```python
from build123d import *

# Parameters (mm, degrees)
F0_R     = 12.7
F0_R_2   = 9.144
F0_R_3   = 2.794
F1_DEPTH = 69.85
F2_DEPTH = 69.851
F3_DEPTH = 19.05


with BuildPart() as f1:
    # F0 (on Top) → F1 (new body)
    with BuildSketch(Plane.XY):
        Circle(F0_R)
        Circle(F0_R_2, mode=Mode.SUBTRACT)
        Circle(F0_R_2)
        Circle(F0_R_3, mode=Mode.SUBTRACT)
        Circle(F0_R_3)
    extrude(amount=F1_DEPTH)

    # F0 (on Top) → F2 (cut, through all)
    with BuildSketch(Plane.XY):
        Circle(F0_R_3)
    extrude(amount=F2_DEPTH, mode=Mode.SUBTRACT)

    # F0 (on Top) → F3 (cut)
    with BuildSketch(Plane.XY):
        Circle(F0_R_2)
        Circle(F0_R_3, mode=Mode.SUBTRACT)
    extrude(amount=F3_DEPTH, mode=Mode.SUBTRACT)


solid = f1.part
```
Can you work these out from the model? Positions are in its coordinate system, mm. A direction names the side the tool comes from. Round coordinates to 2 decimals unless told otherwise and drop trailing zeros. Loops run counter-clockwise (first coordinate to the right, second up) from the corner with the lowest first, then second, coordinate; pieces in that order, holes last.
Item 1: Suppose I cut it at C-C, the plane x = 7.5. Write out the boundary of the cut face in (y, z), then the cut area to 3 significant figures.
Item 2: Will these pins go through, and if not, where does the flat tip stop? pin 1 Ø4 at (x, z) = (9.5, 34.5) entering from +Y; pin 2 Ø4 at (y, z) = (9.5, 51.5) entering from +X; pin 3 Ø1.5 at (y, z) = (-9.5, 15.5) entering from -X.
Item 3: Please list where these lines run through material, in increasing order: L1, parallel to Y at x = 0, z = 7; L2, parallel to Y at x = 0, z = 49; L3, parallel to Z at x = 1, y = 8.5.
Item 4: Which directions (+Z, -Z, +X, -X, +Y, -Y) give clear straight access to the entire face, cutting with the end or side of a thin tool? Please do faces 1 (the cylindrical face through (-2.217, -1.7, 44.094)), 2 (the cylindrical face through (-1.982, -8.927, 9.392)).
Item 5: If we mould it in two halves opening along X, with no side actions, what happens to faces 3 (the flat face through (-9, 3, 0)), 4 (the flat face through (-2.2, 2.2, 19.05)), 5 (the cylindrical face through (-2.75, -12.4, 34.44))? For each: +X half, -X half, draft (parallel to the pull), parting line (faces both ways), or undercut.
Item 6: Suppose I cut it at D-D, the plane z = 49. Write out the boundary of the cut face in (x, y).
Item 7: Suppose I cut it at A-A, the plane y = 0. Write out the boundary of the cut face in (x, z).
Reported:
1. outline: (-10.25, 0) - (-5.23, 0) - (-5.23, 19.05) - (5.23, 19.05) - (5.23, 0) - (10.25, 0) - (10.25, 69.85) - (-10.25, 69.85) - close
1. area: 1,230 mm2
2. pin 1: stops at y = 10.25
2. pin 2: stops at x = 10.25
2. pin 3: stops at x = -9.2
3. L1: y = -12.7 to -9.14, 9.14 to 12.7
3. L2: y = -12.7 to -2.79, 2.79 to 12.7
3. L3: z = 19.05 to 69.85
4. face 1: +Z, -Z
4. face 2: -Z
5. face 3: draft
5. face 4: undercut
5. face 5: parting line
6. outline: circle Ø25.4 at (0, 0); hole circle Ø5.59 at (0, 0)
7. outline: (-12.7, 0) - (-9.14, 0) - (-9.14, 19.05) - (-2.79, 19.05) - (-2.79, 69.85) - (-12.7, 69.85) - close; (2.79, 19.05) - (9.14, 19.05) - (9.14, 0) - (12.7, 0) - (12.7, 69.85) - (2.79, 69.85) - close
